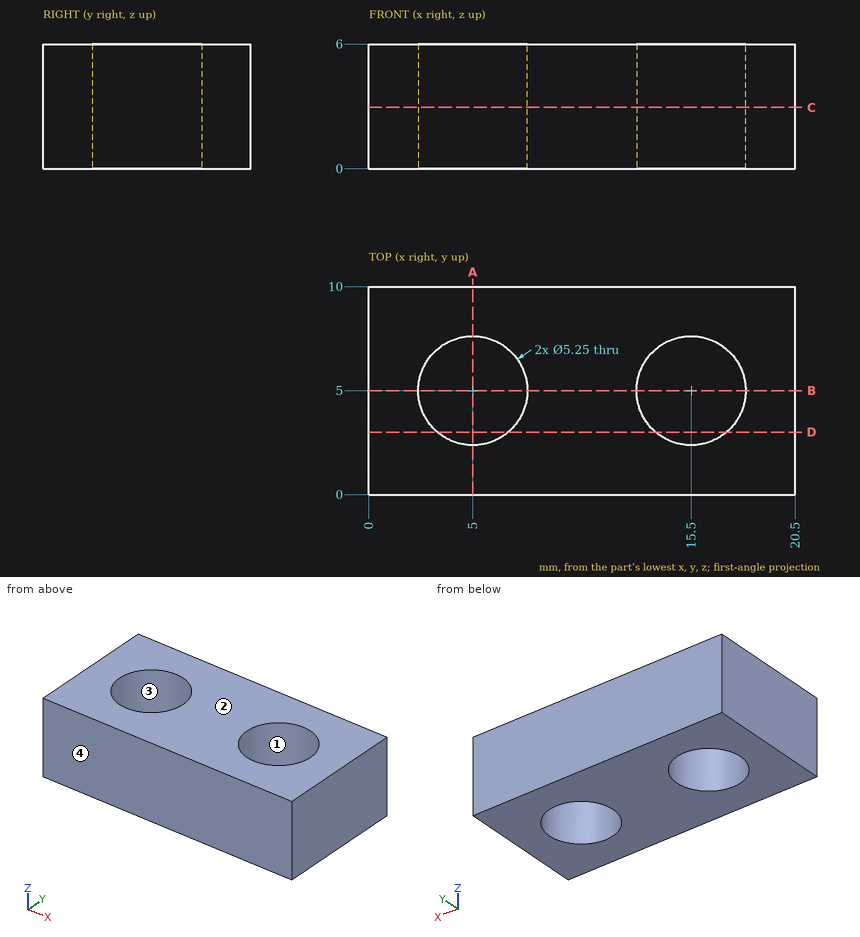
Study the drawing (mm; zero at the part's minimum x, y, z) and answer. Round coordinates to 2 decimals unless told otherwise and drop trailing zeros. Order: outer loops, then holes, each group sorted by start corner. A loop starts at its lowest first (then second) coordinate and runs counter-clockwise, first axis right, second up. Notation, with made-up numbers: (6.5, 58.25) -> (10.5, 58.25) arc R6 ccw to (10.5, 62.25) -> close; hole circle Ø7 at (-26, -5.75). An arc over 180 degrees is marked (long way). Write each question's results on one line, items separated by ' | '. Start each with the question number.
Q1. Find section C-C (z = 2.95). Determine the outline of the cut face in (x, y) (3 decimals), then the cut area to 3 significant figures.
Q2. The mould has two halves that part along Y. Classify the marked faces 1, 2, 3 and 4: pulls with the +Y half, pulls with the -Y half, needs draft (parallel to the pull), parting line crosses it, or undercut.
Q3. Find section B-B (y = 5). Determine the outline of the cut face in (x, z) (3 decimals), then the cut area to 3 significant figures.
Q4. Straight lines are drawn through the part: probe 1 along X at (y, z) = (5, 1.5) (3 decimals); probe 2 along Y at (x, z) = (15.5, 3.5) (3 decimals); probe 3 along X at (y, z) = (4.25, 2.15). For each, find the intervals that lie inside material, in ascending order. Write a range as from..to.
Q5. This flat-tipped pin is pushed along its axis until it touches: pin 1 (4 mm diameter, centred on x = 15.5, y = 5, fed in from +Z). Where does it stop, or does it pass through?
Q6. Find section A-A (x = 5). Determine the outline of the cut face in (y, z) (3 decimals), then the cut area to 3 significant figures.
Q7. Find section D-D (y = 3). Determine the outline of the cut face in (x, z), then the cut area to 3 significant figures.
Worked answers:
1) outline: (0, 0) -> (20.5, 0) -> (20.5, 10) -> (0, 10) -> close; hole circle Ø5.25 at (5, 5); hole circle Ø5.25 at (15.5, 5) | area: 162 mm2
2) face 1: undercut | face 2: needs draft | face 3: undercut | face 4: pulls with the -Y half
3) outline: (0, 0) -> (2.375, 0) -> (2.375, 6) -> (0, 6) -> close; (7.625, 0) -> (12.875, 0) -> (12.875, 6) -> (7.625, 6) -> close; (18.125, 0) -> (20.5, 0) -> (20.5, 6) -> (18.125, 6) -> close | area: 60.0 mm2
4) probe 1: x = 0..2.375, 7.625..12.875, 18.125..20.5 | probe 2: y = 0..2.375, 7.625..10 | probe 3: x = 0..2.48, 7.52..12.98, 18.02..20.5
5) pin 1: passes through
6) outline: (0, 0) -> (2.375, 0) -> (2.375, 6) -> (0, 6) -> close; (7.625, 0) -> (10, 0) -> (10, 6) -> (7.625, 6) -> close | area: 28.5 mm2
7) outline: (0, 0) -> (3.3, 0) -> (3.3, 6) -> (0, 6) -> close; (6.7, 0) -> (13.8, 0) -> (13.8, 6) -> (6.7, 6) -> close; (17.2, 0) -> (20.5, 0) -> (20.5, 6) -> (17.2, 6) -> close | area: 82.2 mm2
